Could you check a few things on this model? Use its own coordinates, in mm. A direction names the side the tool comes from. Round coordinates to 2 decimals unless told otherwise and drop trailing zeros. Loops run counter-clockwise (first coordinate to the right, second up) from the corner with the lowest first, then second, coordinate; pieces in that order, holes last. Notation, with made-up numbers: (-8, 54) - (1, 54) arc R18 ccw to (1, 63) - close; hole circle Ø1 at (-17, 87). An arc over 180 degrees is marked (long way). Use one line per item in the form item = value.
```python
from build123d import *

# Parameters (mm, degrees)
F0_R     = 8.56615
F0_R_2   = 4.826
F1_DEPTH = 32.639
F2_R     = 16.123206
F2_R_2   = 6.31825
F3_DEPTH = 12.0523
F4_R     = 4.826
F5_DEPTH = 6.4008
F6_R     = 5.3594
F7_DEPTH = 8.001


with BuildPart() as f1:
    # F0 (on Top) → F1 (new body)
    with BuildSketch(Plane.XY):
        Circle(F0_R)
        Circle(F0_R_2, mode=Mode.SUBTRACT)
    extrude(amount=F1_DEPTH)

    # F2 (on face) → F3 (cut)
    with BuildSketch(Plane(origin=(0, 0, 0), x_dir=(1, 0, 0), z_dir=(0, 0, -1))):
        Circle(F2_R)
        Circle(F2_R_2, mode=Mode.SUBTRACT)
    extrude(amount=-F3_DEPTH, mode=Mode.SUBTRACT)

    # F4 (on face) → F5 (join)
    with BuildSketch(Plane(origin=(0, 0, 12.0523), x_dir=(1, 0, 0), z_dir=(0, 0, -1))):
        Polygon((5.015326, 8.6868), (-5.015326, 8.6868), (-10.030653, 0), (-5.015326, -8.6868), (5.015326, -8.6868), (10.030653, 0), align=None)
        Circle(F4_R, mode=Mode.SUBTRACT)
    extrude(amount=-F5_DEPTH)

    # F6 (on face) → F7 (cut)
    with BuildSketch(Plane.XY.offset(32.639)):
        Circle(F6_R)
    extrude(amount=-F7_DEPTH, mode=Mode.SUBTRACT)


solid = f1.part
```
1. If we section it at C-C, the plane z = 26: Write out the boundary of the cut face in (x, y), plus the area to 3 significant figures.
Solution:
outline = circle Ø17.13 at (0, 0); hole circle Ø10.72 at (0, 0)
area = 140 mm^2
2. On a 3-axis mill with a long thin cutter (end or side, diameter ignored), from which of +Z, -Z, +X, -X, +Y, -Y can I reach the whole of each face in a straight line? I mean faces 1 (the face through (-7.56, 4.28, 15.21)), 2 (the face through (-6.8, -5.21, 25.45)), 3 (the face through (7, 0, 12.052)). Say none if no direction works.
Solution:
face_1 = +Z, -Z, -X, +Y
face_2 = +Z
face_3 = -Z
3. For P1, Ø10, axis at y = -4, z = 28.5, coming from the +X side; P2, Ø5.5, axis at x = -2, y = 1.5, coming from the +Z side; P3, Ø6, axis at x = -0.5, z = 27, coming from the +Y side, each with a flat end and sliding along its axis, tell me the tip position at first contact or that it passes through.
Solution:
P1 = 8.57
P2 = 24.64
P3 = 8.57
4. If we section it at A-A, the plane x = 0: Write out the boundary of the cut face in (y, z), plus the area to 3 significant figures.
Solution:
outline = (-8.69, 12.05) - (-6.32, 12.05) - (-6.32, 0) - (-4.83, 0) - (-4.83, 24.64) - (-5.36, 24.64) - (-5.36, 32.64) - (-8.57, 32.64) - (-8.57, 18.45) - (-8.69, 18.45) - close; (4.83, 0) - (6.32, 0) - (6.32, 12.05) - (8.69, 12.05) - (8.69, 18.45) - (8.57, 18.45) - (8.57, 32.64) - (5.36, 32.64) - (5.36, 24.64) - (4.83, 24.64) - close
area = 183 mm^2
5. We'd pull the mould along Y, two halves only. Please class faces 4 (the face through (-5, 1, 24.638)), 5 (the face through (-7.49, -4.4, 15.21)), 6 (the face through (-3.83, -2.937, 12.147)), 7 (the face through (-1, -5, 0)): +Y half, -Y half, draft (parallel to the pull), parting line (faces both ways), or undercut.
Solution:
face_4 = undercut
face_5 = -Y half
face_6 = undercut
face_7 = draft
6. Please list where these lines run through material, in increasing order: line 1 along X through (y, z) = (0, 6.5); line 2 along Y through (x, z) = (0, 30.75).
Solution:
line_1 = -6.32 to -4.83, 4.83 to 6.32
line_2 = -8.57 to -5.36, 5.36 to 8.57
7. If we section it at B-B, the plane y = -1.5: Write out the boundary of the cut face in (x, z), plus the area to 3 significant figures.
Solution:
outline = (-9.16, 12.05) - (-6.14, 12.05) - (-6.14, 0) - (-4.59, 0) - (-4.59, 24.64) - (-5.15, 24.64) - (-5.15, 32.64) - (-8.43, 32.64) - (-8.43, 18.45) - (-9.16, 18.45) - close; (4.59, 0) - (6.14, 0) - (6.14, 12.05) - (9.16, 12.05) - (9.16, 18.45) - (8.43, 18.45) - (8.43, 32.64) - (5.15, 32.64) - (5.15, 24.64) - (4.59, 24.64) - close
area = 196 mm^2
8. If we section it at D-D, the plane x = 7.25: Write out the boundary of the cut face in (y, z).
Solution:
outline = (-4.82, 12.05) - (4.82, 12.05) - (4.82, 18.45) - (4.56, 18.45) - (4.56, 32.64) - (-4.56, 32.64) - (-4.56, 18.45) - (-4.82, 18.45) - close
